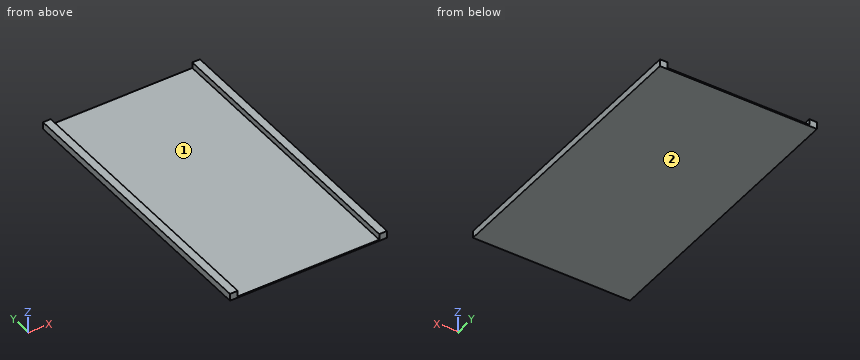
```python
from build123d import *

# Parameters (mm, degrees)
F0_W     = 127
F0_H     = 2.221532
F1_DEPTH = 508


with BuildPart() as f1:
    # F0 (on Front) → F1 (new body)
    with BuildSketch(Plane.XZ):
        with Locations((63.5, 0)):
            Rectangle(F0_W, F0_H)
        Polygon((127, 1.110766), (127, -1.110766), (140.89732, -1.110766), (140.89732, 11.589234), (127, 11.589234), align=None)
        with Locations((-63.5, 0)):
            Rectangle(F0_W, F0_H)
        Polygon((-140.89732, -1.110766), (-127, -1.110766), (-127, 1.110766), (-127, 11.589234), (-140.89732, 11.589234), align=None)
    extrude(amount=F1_DEPTH)


solid = f1.part
```
Work out the finished part from the listing and answer in its coordinate system (mm). Face numbers are marked on the shaded views. Give positions to 0.01 mm unless a question says otherwise; leave off trailing zeros. Loops run counter-clockwise (first coordinate to the right, second up) from the corner with the lowest first, then second, coordinate; pieces in that order, holes last. Notation, with made-up numbers: (-26.5, 16.5) - (15.5, 16.5) arc R12 ccw to (15.5, 28.5) - close; hole circle Ø9 at (-39.75, 40.5). An arc over 180 degrees is marked (long way). One line per question, with ' | ' between items.
(1) This flat-tipped pin is pushed along its axis until it touches: pin 1 Ø4 at (x, y) = (35.5, -228) entering from +Z. Where does it stop, or does it pass through?
Recorded:
pin 1: stops at z = 1.11
(2) The part is cut by section B-B (y = -262.5). Write down the section's boundary in (x, z).
Recorded:
outline: (-140.9, -1.11) - (140.9, -1.11) - (140.9, 11.59) - (127, 11.59) - (127, 1.11) - (-127, 1.11) - (-127, 11.59) - (-140.9, 11.59) - close
(3) Straight lines are drawn through the part: probe 1 along X at (y, z) = (-168.5, 4.25); probe 2 along Z at (x, y) = (-2, -365). For each, find the intervals that lie inside material, in ascending order.
Recorded:
probe 1: x = -140.9 to -127, 127 to 140.9 | probe 2: z = -1.11 to 1.11
(4) The part is cut by section C-C (x = -78). Write down the section's boundary in (y, z), then the cut area to 3 significant figures.
Recorded:
outline: (-508, -1.11) - (0, -1.11) - (0, 1.11) - (-508, 1.11) - close | area: 1,130 mm²
(5) The part is cut by section A-A (z = 6.75). Write down the section's boundary in (x, y).
Recorded:
outline: (-140.9, -508) - (-127, -508) - (-127, 0) - (-140.9, 0) - close; (127, -508) - (140.9, -508) - (140.9, 0) - (127, 0) - close
(6) The mould has two halves that part along X. Classify the marked faces 1 and 2: +X half, -X half, draft (parallel to the pull), parting line (faces both ways), or undercut.
Recorded:
face 1: undercut | face 2: draft
